Build history of the part. All positions in model axes, mm. A direction names the side the tool comes from. Round coordinates to 2 decimals unless told otherwise and drop trailing zeros. Loops run counter-clockwise (first coordinate to the right, second up) from the corner with the lowest first, then second, coordinate; pieces in that order, holes last.
from build123d import *

# Parameters (mm, degrees)
SKETCH1_W           = 19.05
SKETCH1_H           = 25.4
BOSS_EXTRUDE1_DEPTH = 38.1
SKETCH2_R           = 4.7625
CUT_EXTRUDE1_DEPTH  = 26.4
SKETCH3_R           = 6.1595
CUT_EXTRUDE2_DEPTH  = 20.05
CUT_EXTRUDE3_REACH  = 40.1
SKETCH4_R           = 2.3495
SKETCH5_R           = 2.3495
CUT_EXTRUDE4_DEPTH  = 26.4


with BuildPart() as part:
    # Sketch1 → Boss-Extrude1 (new body)
    with BuildSketch(Plane(origin=(0, 0, 0), x_dir=(1, 0, 0), z_dir=(0, 1, 0))):
        Rectangle(SKETCH1_W, SKETCH1_H)
    extrude(amount=BOSS_EXTRUDE1_DEPTH)

    # Sketch2 → Cut-Extrude1 (cut, through all)
    with BuildSketch(Plane.XY.offset(12.7)):
        with Locations((0, 7.9375)):
            Circle(SKETCH2_R)
    extrude(amount=-CUT_EXTRUDE1_DEPTH, mode=Mode.SUBTRACT)

    # Sketch3 → Cut-Extrude2 (cut, through all)
    with BuildSketch(Plane(origin=(9.525, 0, 0), x_dir=(0, 0, -1), z_dir=(1, 0, 0))):
        with Locations((0, 25.654)):
            Circle(SKETCH3_R)
    extrude(amount=-CUT_EXTRUDE2_DEPTH, mode=Mode.SUBTRACT)

    # Sketch4 → Cut-Extrude3 (cut, up to next)
    with BuildSketch(Plane(origin=(0, 38.1, 0), x_dir=(1, 0, 0), z_dir=(0, 1, 0)), mode=Mode.PRIVATE) as cut_extrude3_sk1:
        Circle(SKETCH4_R)
    cut_extrude3_tool1 = extrude(cut_extrude3_sk1.sketch, amount=-CUT_EXTRUDE3_REACH, mode=Mode.PRIVATE) & part.part
    add(cut_extrude3_tool1.solids().sort_by_distance((0, 38.1, 0))[0], mode=Mode.SUBTRACT)

    # Sketch5 → Cut-Extrude4 (cut, through all)
    with BuildSketch(Plane(origin=(0, 0, -12.7), x_dir=(-1, 0, 0), z_dir=(0, 0, -1))):
        with Locations((0, 25.4)):
            Circle(SKETCH5_R)
    extrude(amount=-CUT_EXTRUDE4_DEPTH, mode=Mode.SUBTRACT)


solid = part.part
(1) Which spindle directions (+Z, -Z, +X, -X, +Y, -Y) get a long thin tool onto all of the face, cutting with end or side? Do faces 1 (the face through (-0.509, 34.771, 2.294)), 2 (the face through (0.13, 20.19, -2.84)). Say none if no direction does.
Responses:
face 1: +Y
face 2: +X, -X
(2) Pin check, flat tip, straight feed: P1, Ø11, axis at y = 25.654, z = 0, coming from the -X side. Stop position of the tip, or through.
Responses:
P1: passes through
(3) Pull direction X, two halves, no side cores. Call faces 3 (the face through (9.525, 19, 0)), 4 (the face through (-9.525, 19, 0)), 5 (the face through (0, 19, -12.7)), 6 (the face through (2.347, 25.503, -9.191)): +X half, -X half, draft (parallel to the pull), parting line (faces both ways), or undercut.
Responses:
face 3: +X half
face 4: -X half
face 5: draft
face 6: undercut
(4) Slice it at A-A on z = -4. List the corners of the cut face in (x, y) (1 decimal).
Responses:
outline: (-9.5, 0) - (9.5, 0) - (9.5, 21) - (-9.5, 21) - close; (-9.5, 30.3) - (9.5, 30.3) - (9.5, 38.1) - (-9.5, 38.1) - close; hole circle Ø9.5 at (0, 7.9)
(5) Slice it at C-C on y = 11. List the corners of the cut face in (x, z) (3 decimals), plus the area to 3 significant figures.
Responses:
outline: (-9.525, -12.7) - (-3.647, -12.7) - (-3.647, 12.7) - (-9.525, 12.7) - close; (3.647, -12.7) - (9.525, -12.7) - (9.525, 12.7) - (3.647, 12.7) - close
area: 299 mm2
(6) Probe line 1 (Z direction, x = -6, y = 25.5); line 2 (X direction, y = 25.4, z = -7) (1 decimal); line 3 (Y direction, x = 1.75, z = -10.25). List the from-to ranges inside material, lowest first.
Responses:
line 1: z = -12.7 to -6.16, 6.16 to 12.7
line 2: x = -9.5 to -2.3, 2.3 to 9.5
line 3: y = 0 to 3.51, 12.37 to 23.83, 26.97 to 38.1
(7) Slice it at B-B on x = 0. List the corners of the cut face in (y, z) (1 decimal), plus the area to 3 significant figures.
Responses:
outline: (0, -12.7) - (3.2, -12.7) - (3.2, 12.7) - (0, 12.7) - close; (12.7, -12.7) - (23.1, -12.7) - (23.1, -5.6) arc R6.2 cw to (23.1, 5.6) - (23.1, 12.7) - (12.7, 12.7) - close; (27.7, -12.7) - (38.1, -12.7) - (38.1, -2.3) - (31.3, -2.3) arc R6.2 cw to (27.7, -5.8) - close; (27.7, 5.8) arc R6.2 cw to (31.3, 2.3) - (38.1, 2.3) - (38.1, 12.7) - (27.7, 12.7) - close
area: 513 mm2
(8) Slice it at D-D on z = 0. List the corners of the cut face in (x, y) (1 decimal), plus the area to 3 significant figures.
Responses:
outline: (-9.5, 0) - (9.5, 0) - (9.5, 19.5) - (-9.5, 19.5) - close; (-9.5, 31.8) - (-2.3, 31.8) - (-2.3, 38.1) - (-9.5, 38.1) - close; (2.3, 31.8) - (9.5, 31.8) - (9.5, 38.1) - (2.3, 38.1) - close; hole circle Ø9.5 at (0, 7.9)
area: 390 mm2
